The listing builds one solid part. Answer for the finished solid, in the listing's coordinates (mm). A direction names the side the tool comes from. Coordinates: 2 decimals unless noted, no trailing zeros. Loops run counter-clockwise (first coordinate to the right, second up) from the corner with the lowest first, then second, coordinate; pieces in that order, holes last. Notation, with made-up numbers: (-28.5, 41) - (-20.5, 41) arc R6 cw to (-20.5, 52) - close; hole circle Ø2 at (0, 51). An arc over 180 degrees is marked (long way). Return JSON: item names as keys, results as strings. Group by question number.
1. The mould has two halves that part along X. Classify faces 1 (the face through (-14.524, -13.632, -5.121)), 2 (the face through (17, 0, -11)), 3 (the face through (0, 28.3, -9)): pulls with the +X half, pulls with the -X half, needs draft (parallel to the pull), parting line crosses it, or undercut.
2. Section A-A (z = -9) is taken. Write down the section's boundary in (x, y), and give its area (3 significant figures).
3. Which of the six approach directions +Z, -Z, +X, -X, +Y, -Y give full straight-line access (tool end or side, diameter ignored) to faces 4 (the face through (-7.5, 0, -18)), 5 (the face through (-14.524, 12.368, -5.121)), 6 (the face through (12, 0, -23.3))?
4. Each of these flat-tipped pins is pushed along its axis until it touches: P1, Ø3, axis at x = -13, y = 13, coming from the +Z side; P2, Ø1, axis at x = 6.5, z = -20, coming from the -Y side; P3, Ø1.5, axis at x = -0.5, y = -4.5, coming from the -Z side; P4, Ø2.5, axis at x = 13, y = -13, coming from the +Z side. Where does it stop, or does it pass through?
5. Section C-C (y = 3) is taken. Write down the section's boundary in (x, z).
6. Find the intervals of material crossed by line 1 along X through (y, z) = (-13, -5.25); line 2 along Y through (x, z) = (-13, -2.25); line 3 along X through (y, z) = (-4.5, -15.5), in increasing order.
7. Section B-B (z = -14.5) is taken. Write down the section's boundary in (x, y), and give its area (3 significant figures).
```python
from build123d import *

# Parameters (mm, degrees)
SKETCH_1_W          = 34
SKETCH_1_H          = 23.3
EXTRUDE_1_DEPTH     = 28.3
SKETCH_2_W          = 15
SKETCH_2_H          = 10.3
CUT_EXTRUDE_1_DEPTH = 64.525191853
M4X0_7_1_D          = 3.3
M4X0_7_1_DEPTH      = 10.1
M4X0_7_1_TIP        = 0.991420021


with BuildPart() as part:
    # 草图1 → 凸台-拉伸1 (new, symmetric)
    with BuildSketch(Plane(origin=(0, 0, 0), x_dir=(1, 0, 0), z_dir=(0, 1, 0))):
        with Locations((0, 11.65)):
            Rectangle(SKETCH_1_W, SKETCH_1_H)
    extrude(amount=EXTRUDE_1_DEPTH, both=True)

    # 草图2 → 切除-拉伸1 (cut, through all)
    with BuildSketch(Plane(origin=(0, 28.3, 0), x_dir=(1, 0, 0), z_dir=(0, 1, 0))):
        with Locations((0, 18.15)):
            Rectangle(SKETCH_2_W, SKETCH_2_H)
    extrude(amount=-CUT_EXTRUDE_1_DEPTH, mode=Mode.SUBTRACT)

    # M4x0.7 螺纹孔1
    with Locations(Plane.XY):
        with Locations((-13, 13), (-13, -13), (13, -13), (13, 13)):
            Hole(M4X0_7_1_D / 2, depth=M4X0_7_1_DEPTH)
            with Locations((0, 0, -(M4X0_7_1_DEPTH + M4X0_7_1_TIP / 2))):  # 118° drill point
                Cone(0, M4X0_7_1_D / 2, M4X0_7_1_TIP, mode=Mode.SUBTRACT)


solid = part.part
```
The answers:
{
 "1": {"face 1": "undercut", "face 2": "pulls with the +X half", "face 3": "needs draft"},
 "2": {"outline": "(-17, -28.3) - (17, -28.3) - (17, 28.3) - (-17, 28.3) - close; hole circle Ø3.3 at (-13, -13); hole circle Ø3.3 at (-13, 13); hole circle Ø3.3 at (13, -13); hole circle Ø3.3 at (13, 13)", "area": "1,890 mm2"},
 "3": {"face 4": "-Z, +Y, -Y", "face 5": "+Z", "face 6": "-Z, +X, -X, +Y, -Y"},
 "4": {"P1": "stops at z = -10.19", "P2": "passes through", "P3": "stops at z = -13", "P4": "stops at z = -10.34"},
 "5": {"outline": "(-17, -23.3) - (-7.5, -23.3) - (-7.5, -13) - (7.5, -13) - (7.5, -23.3) - (17, -23.3) - (17, 0) - (-17, 0) - close"},
 "6": {"line 1": "x = -17 to -14.65, -11.35 to 11.35, 14.65 to 17", "line 2": "y = -28.3 to -14.65, -11.35 to 11.35, 14.65 to 28.3", "line 3": "x = -17 to -7.5, 7.5 to 17"},
 "7": {"outline": "(-17, -28.3) - (-7.5, -28.3) - (-7.5, 28.3) - (-17, 28.3) - close; (7.5, -28.3) - (17, -28.3) - (17, 28.3) - (7.5, 28.3) - close", "area": "1,080 mm2"}
}
